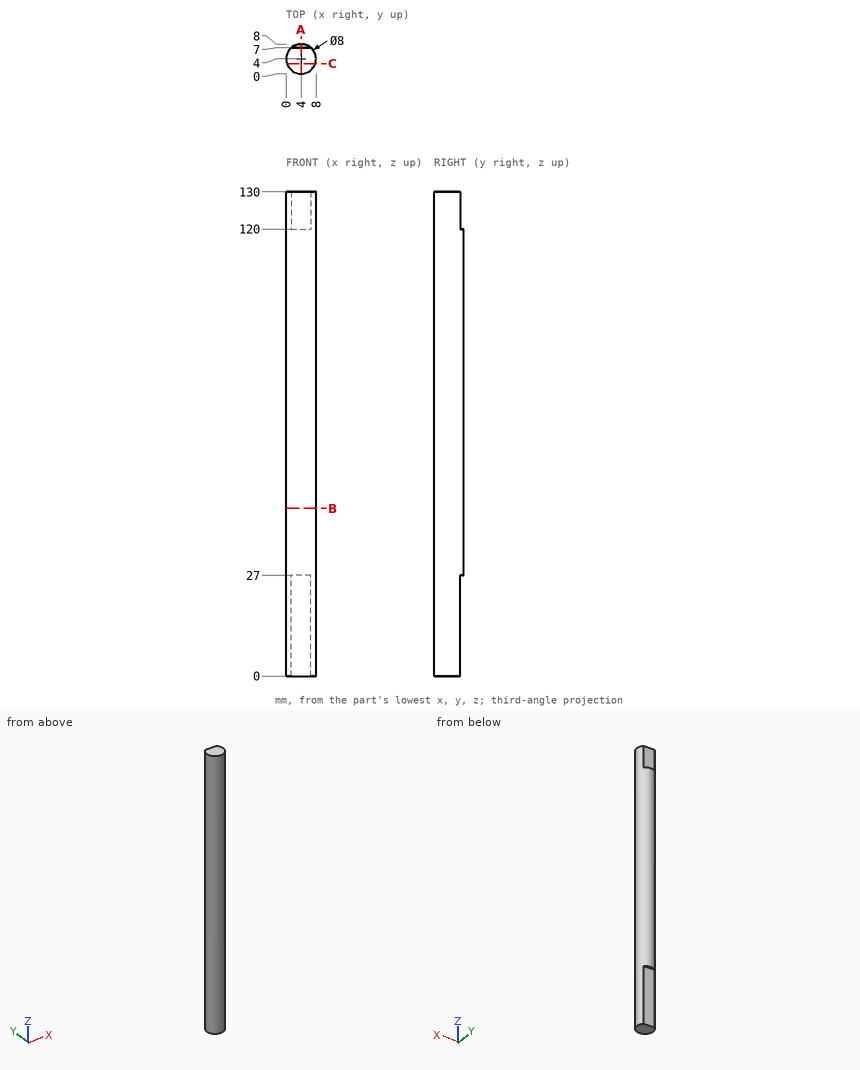
Can you work these out from the drawing? Everything is in mm from the part's minimum corner. Round coordinates to 2 decimals unless told otherwise and drop trailing zeros. Write each loop counter-clockwise with the first axis right and the second up, starting at its lowest first coordinate (ties: lowest second). Pieces come first, ordered by that corner, then holes. Notation, with made-up numbers: (66, 22) - (94, 22) arc R7 cw to (94, 28) - close; hole circle Ø9 at (9, 76.25). An arc over 180 degrees is marked (long way). Put each result on its own line as item: value. Start each with the question number.
(1) I need wall thicknesses on probe 1 along X at (y, z) = (4.25, 42.5); probe 2 along X at (y, z) = (7, 60). Which ranges of each line are inside material? Lowest first, please.
(2) I want a section at A-A, the plane x = 4. Please give me the cut outline in (y, z), plus the area to 3 significant figures.
(3) Will these pins go through, and if not, where does the flat tip stop? pin 1 (1 mm diameter, centred on x = 2.5, z = 36.5, fed in from -Y); pin 2 (3 mm diameter, centred on y = 2, z = 22, fed in from -X); pin 3 (1.5 mm diameter, centred on x = 7, z = 16, fed in from +Y).
(4) I want a section at B-B, the plane z = 45. Please give me the cut outline in (x, y), plus the area to 3 significant figures.
(5) I want a section at C-C, the plane y = 2.75. Please give me the cut outline in (x, z), plus the area to 3 significant figures.
Here are the results:
1. probe 1: x = 0.01 to 7.99
1. probe 2: x = 1.35 to 6.65
2. outline: (0, 0) - (7, 0) - (7, 27) - (8, 27) - (8, 120) - (7, 120) - (7, 130) - (0, 130) - close
2. area: 1,000 mm^2
3. pin 1: stops at y = 0.13
3. pin 2: stops at x = 0.03
3. pin 3: stops at y = 7
4. outline: circle Ø8 at (4, 4)
4. area: 50.3 mm^2
5. outline: (0.2, 0) - (7.8, 0) - (7.8, 130) - (0.2, 130) - close
5. area: 988 mm^2
